CAD build for the part. Positions are in the model's coordinates, mm. Face numbers are marked on the shaded views. A direction names the side the tool comes from. Round coordinates to 2 decimals unless told otherwise and drop trailing zeros. Write each loop counter-clockwise with the first axis right and the second up, starting at its lowest first coordinate (ties: lowest second). Pieces come first, ordered by that corner, then holes. Notation, with made-up numbers: (55.5, 7) - (72.5, 7) arc R18 ccw to (72.5, 16) - close; hole circle Ø4 at (15, 68). An arc over 180 degrees is marked (long way). Answer in a Markdown table with one row per item.
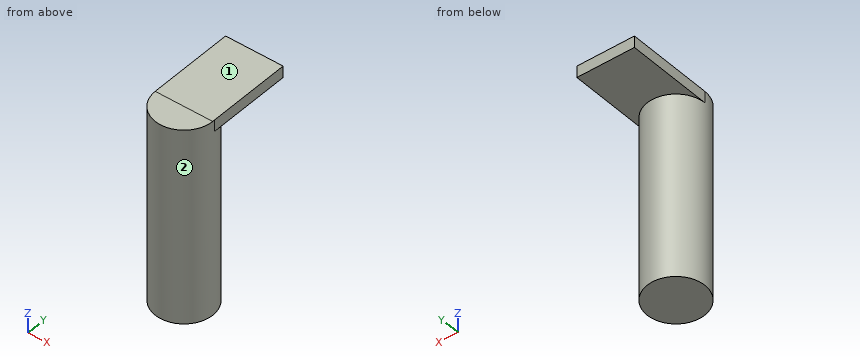
```python
from build123d import *

# Parameters (mm, degrees)
SKETCH1_R           = 5
BOSS_EXTRUDE1_DEPTH = 34
SKETCH3_W           = 10
SKETCH3_H           = 2
BOSS_EXTRUDE2_DEPTH = 15


with BuildPart() as part:
    # Sketch1 → Boss-Extrude1 (new body)
    with BuildSketch(Plane.XY):
        with Locations((-14.936060675, 10.217847077)):
            Circle(SKETCH1_R)
    extrude(amount=BOSS_EXTRUDE1_DEPTH)

    # Sketch3 → Boss-Extrude2 (add)
    with BuildSketch(Plane(origin=(-0.118548513, 10.386962355, 0), x_dir=(0.999934876, 0.01141246, 0), z_dir=(-0.01141246, 0.999934876, 0))):
        with Locations((-14.829416568, -33.000036039)):
            Rectangle(SKETCH3_W, SKETCH3_H)
    extrude(amount=BOSS_EXTRUDE2_DEPTH)


solid = part.part
```
Q1. Drill centre lines: line 1 (Z direction, x = -14.75, y = 19.5); line 2 (Y direction, x = -16, z = 12); line 3 (Y direction, x = -18.5, z = 15). Where is each one in solid material? Low to high.
Computed:
| item | result |
|---|---|
| line 1 | z = 32 to 34 |
| line 2 | y = 5.33 to 15.1 |
| line 3 | y = 6.71 to 13.72 |
Q2. Saw through at D-D on y = 20.75. List the corners of the cut face in (x, z), then the cut area to 3 significant figures.
Computed:
| item | result |
|---|---|
| outline | (-20.07, 32) - (-10.07, 32) - (-10.07, 34) - (-20.07, 34) - close |
| area | 20.0 mm2 |
Q3. Saw through at A-A on y = 11.5. List the corners of the cut face in (x, z).
Computed:
| item | result |
|---|---|
| outline | (-19.96, 32) - (-19.77, 32) - (-19.77, 0) - (-10.1, 0) - (-10.1, 32) - (-9.96, 32) - (-9.96, 34) - (-19.96, 34) - close |
Q4. 3-axis set-ups, long thin cutter, end or side, ignore diameter. For the marked faces 1 and 2: which of +Z, -Z, +X, -X, +Y, -Y reach the whole face in a straight line?
Computed:
| item | result |
|---|---|
| face 1 | +Z, +X, -X, +Y, -Y |
| face 2 | -Z |
Q5. Saw through at C-C on z = 7. List the corners of the cut face in (x, y), then the cut area to 3 significant figures.
Computed:
| item | result |
|---|---|
| outline | circle Ø10 at (-14.94, 10.22) |
| area | 78.5 mm2 |
Q6. Flat gauge pins, fed straight in: pin 1 (6 mm diameter, centred on x = -18.5, z = 28, fed in from +Y); pin 2 (5 mm diameter, centred on x = -11, z = 26, fed in from -Y). Where does each tip first touch, or does it go through?
Computed:
| item | result |
|---|---|
| pin 1 | stops at y = 15.19 |
| pin 2 | stops at y = 5.43 |
